Verification items for the finished model (mm, model axes). Give positions to 0.01 mm unless a question says otherwise; leave off trailing zeros. Loops run counter-clockwise (first coordinate to the right, second up) from the corner with the lowest first, then second, coordinate; pieces in that order, holes last. Notation, with made-up numbers: M 69.25,17 L 122.25,17 A24 ccw 122.25,37 Z; hole C 69,21.5 d5. An arc over 180 degrees is marked long. Write each question's results on one line, items separated by ' | '. Start each with the question number.
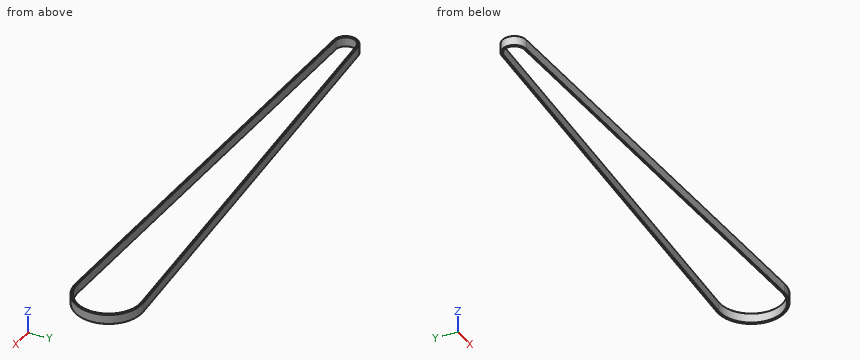
Autodesk Inventor part; units mm, degrees
ref_plane "YZ Plane" through (0, 0, 0) normal (1, 0, 0) x (0, 1, 0)
ref_plane "XZ Plane" through (0, 0, 0) normal (0, 1, 0) x (-1, 0, 0)
ref_plane "XY Plane" through (0, 0, 0) normal (0, 0, 1) x (1, 0, 0)
sketch "Sketch1" plane through (0, 0, 0) normal (0, 0, 1) x (1, 0, 0)
  arc A0 (-0.2852, 5.9932) -> (-0.2852, -5.9932) centre (0, 0) ccw
  arc A1 (269.4505, -18.8287) -> (269.4505, 18.8287) centre (270.3465, 0) ccw
  line L0 (269.4505, 18.8287) -> (-0.2852, 5.9932)
  line L1 (-0.2852, -5.9932) -> (269.4505, -18.8287)
  line L2 (-0.347, 7.2917) -> (269.3887, 20.1272)
  arc A2 (269.3887, -20.1272) -> (269.3887, 20.1272) centre (270.3465, 0) ccw
  line L3 (269.3887, -20.1272) -> (-0.347, -7.2917)
  arc A3 (-0.347, 7.2917) -> (-0.347, -7.2917) centre (0, 0) ccw
  dimension "d0" = 12
  dimension "d1" = 37.7
  dimension "d3" = 1.3
  dimension "d9" = 270.3465
extrude "Extrusion1" add sketch "Sketch1" along normal mid plane 6
chamfer "Chamfer1" distance 0.2 angle 45 16 edges at (289.1965, 0, 3) (134.5826, -12.411, 3) (-6, 0, 3) (134.5826, 12.411, 3) (289.1965, 0, -3) (134.5826, 12.411, -3) (-6, 0, -3) (134.5826, -12.411, -3) (290.4965, 0, 3) (134.5209, 13.7095, 3) (-7.3, 0, 3) (134.5209, -13.7095, 3) (290.4965, 0, -3) (134.5209, -13.7095, -3) (-7.3, 0, -3) (134.5209, 13.7095, -3)
properties part number "Tandriem20naar60T-696mm" material "Rubber"
1. Section check A-A, the plane z = 1.25. Record the boundary of the cut face in (x, y), plus the area to 3 significant figures.
2. Depth check by flat-ended pin: pin 1 Ø2 at (x, z) = (83.5, 2.5) entering from +Y; pin 2 Ø3 at (x, z) = (111, 0) entering from -Y. Enter the tip coordinate at first touch or a pass-through.
3. Thickness scan on probe 1 along Y at (x, z) = (30, -1.25); probe 2 along Y at (x, z) = (166, -1); probe 3 along X at (y, z) = (4.5, 1.75). Record the ranges inside material, lowest first.
4. Section check B-B, the plane y = 0. Record the boundary of the cut face in (x, z), plus the area to 3 significant figures.
5. Section check C-C, the plane x = 246. Record the boundary of the cut face in (y, z), plus the area to 3 significant figures.
Filled sheet:
1) outline: M -0.35,-7.29 L 269.39,-20.13 A20.15 ccw long 269.39,20.13 L -0.35,7.29 A7.3 ccw Z; hole M -0.29,-5.99 L 269.45,-18.83 A18.85 ccw long 269.45,18.83 L -0.29,5.99 A6 ccw Z | area: 810 mm2
2) pin 1: y = 11.33 | pin 2: y = -12.66
3) probe 1: -8.74 to -7.43, 7.43 to 8.74 | probe 2: -15.21 to -13.91, 13.91 to 15.21 | probe 3: -5.75 to -3.97, 288.65 to 289.99
4) outline: M -7.3,-2.8 L -7.1,-3 L -6.2,-3 L -6,-2.8 L -6,2.8 L -6.2,3 L -7.1,3 L -7.3,2.8 Z; M 289.2,-2.8 L 289.4,-3 L 290.3,-3 L 290.5,-2.8 L 290.5,2.8 L 290.3,3 L 289.4,3 L 289.2,2.8 Z | area: 15.4 mm2
5) outline: M -19.01,-2.8 L -18.81,-3 L -17.91,-3 L -17.71,-2.8 L -17.71,2.8 L -17.91,3 L -18.81,3 L -19.01,2.8 Z; M 17.71,-2.8 L 17.91,-3 L 18.81,-3 L 19.01,-2.8 L 19.01,2.8 L 18.81,3 L 17.91,3 L 17.71,2.8 Z | area: 15.5 mm2
